from build123d import *

# Parameters (mm, degrees)
F0_R      = 30
F0_R_2    = 27.5
F1_DEPTH  = 38
F3_R      = 30
F3_R_2    = 27.5
F4_DEPTH  = 40
F6_W      = 24
F6_H      = 32
F7_DEPTH  = 65
F9_DEPTH  = 24
F10_DEPTH = 38
F12_DEPTH = 38
F13_R     = 4
F14_DEPTH = 38


with BuildPart() as f1:
    # F0 (on Front) → F1 (new body)
    with BuildSketch(Plane.XZ):
        with BuildLine():
            ThreePointArc((-32.5, 26.5), (-28.2573593129, 28.2573593129), (-26.5, 32.5))
            Line((-26.5, 32.5), (-28.5, 32.5))
            ThreePointArc((-28.5, 32.5), (-29.6715728753, 29.6715728753), (-32.5, 28.5))
            Line((-32.5, 28.5), (-32.5, 26.5))
        make_face()
        with BuildLine():
            Line((-28.5, 32.5), (-26.5, 32.5))
            ThreePointArc((-26.5, 32.5), (-36.7426406871, 36.7426406871), (-32.5, 26.5))
            Line((-32.5, 26.5), (-32.5, 28.5))
            ThreePointArc((-32.5, 28.5), (-35.3284271247, 35.3284271247), (-28.5, 32.5))
        make_face()
        with BuildLine():
            Line((26.5, 32.5), (-26.5, 32.5))
            ThreePointArc((-26.5, 32.5), (-28.2573593129, 28.2573593129), (-32.5, 26.5))
            Line((-32.5, 26.5), (-32.5, -26.5))
            ThreePointArc((-32.5, -26.5), (-28.2573593129, -28.2573593129), (-26.5, -32.5))
            Line((-26.5, -32.5), (26.5, -32.5))
            ThreePointArc((26.5, -32.5), (28.2573593129, -28.2573593129), (32.5, -26.5))
            Line((32.5, -26.5), (32.5, 26.5))
            ThreePointArc((32.5, 26.5), (28.2573593129, 28.2573593129), (26.5, 32.5))
        make_face()
        Circle(F0_R, mode=Mode.SUBTRACT)
        with BuildLine():
            ThreePointArc((38.5, 32.5), (32.5, 38.5), (26.5, 32.5))
            Line((26.5, 32.5), (28.5, 32.5))
            ThreePointArc((28.5, 32.5), (32.5, 36.5), (36.5, 32.5))
            ThreePointArc((36.5, 32.5), (35.3284271247, 29.6715728753), (32.5, 28.5))
            Line((32.5, 28.5), (32.5, 26.5))
            ThreePointArc((32.5, 26.5), (36.7426406871, 28.2573593129), (38.5, 32.5))
        make_face()
        with BuildLine():
            Line((28.5, 32.5), (26.5, 32.5))
            ThreePointArc((26.5, 32.5), (28.2573593129, 28.2573593129), (32.5, 26.5))
            Line((32.5, 26.5), (32.5, 28.5))
            ThreePointArc((32.5, 28.5), (29.6715728753, 29.6715728753), (28.5, 32.5))
        make_face()
        with BuildLine():
            ThreePointArc((-26.5, -32.5), (-28.2573593129, -28.2573593129), (-32.5, -26.5))
            Line((-32.5, -26.5), (-32.5, -28.5))
            ThreePointArc((-32.5, -28.5), (-29.6715728753, -29.6715728753), (-28.5, -32.5))
            Line((-28.5, -32.5), (-26.5, -32.5))
        make_face()
        with BuildLine():
            Line((-32.5, -28.5), (-32.5, -26.5))
            ThreePointArc((-32.5, -26.5), (-36.7426406871, -36.7426406871), (-26.5, -32.5))
            Line((-26.5, -32.5), (-28.5, -32.5))
            ThreePointArc((-28.5, -32.5), (-35.3284271247, -35.3284271247), (-32.5, -28.5))
        make_face()
        with BuildLine():
            ThreePointArc((38.5, -32.5), (36.7426406871, -28.2573593129), (32.5, -26.5))
            Line((32.5, -26.5), (32.5, -28.5))
            ThreePointArc((32.5, -28.5), (35.3284271247, -29.6715728753), (36.5, -32.5))
            ThreePointArc((36.5, -32.5), (32.5, -36.5), (28.5, -32.5))
            Line((28.5, -32.5), (26.5, -32.5))
            ThreePointArc((26.5, -32.5), (32.5, -38.5), (38.5, -32.5))
        make_face()
        with BuildLine():
            Line((32.5, -28.5), (32.5, -26.5))
            ThreePointArc((32.5, -26.5), (28.2573593129, -28.2573593129), (26.5, -32.5))
            Line((26.5, -32.5), (28.5, -32.5))
            ThreePointArc((28.5, -32.5), (29.6715728753, -29.6715728753), (32.5, -28.5))
        make_face()
        Circle(F0_R)
        Circle(F0_R_2, mode=Mode.SUBTRACT)
    extrude(amount=F1_DEPTH)

    # F3 (on offset) → F4 (join)
    with BuildSketch(Plane.XZ.offset(1)):
        Circle(F3_R)
        Circle(F3_R_2, mode=Mode.SUBTRACT)
    extrude(amount=-F4_DEPTH)

    # F6 (on offset) → F7 (join)
    with BuildSketch(Plane.XY.offset(-32.5)):
        with Locations((-44.5, -22)):
            Rectangle(F6_W, F6_H)
    extrude(amount=F7_DEPTH)

    # F8 (on face) → F9 (cut)
    with BuildSketch(Plane(origin=(-56.5, 0, 0), x_dir=(0, -1, 0), z_dir=(-1, 0, 0))):
        with BuildLine():
            Line((11.5996693186, -18.5), (6, -18.5))
            Line((6, -18.5), (6, -32.5))
            Line((6, -32.5), (19.7712382075, -32.5))
            ThreePointArc((19.7712382075, -32.5), (17.3473955456, -31.8732124062), (15.5312466875, -30.1499947))
            Line((15.5312466875, -30.1499947), (12.76000848, -25.716013568))
            ThreePointArc((12.76000848, -25.716013568), (12.1937562692, -24.4444314332), (12, -23.0660188679))
            Line((12, -23.0660188679), (12, -18.9003306814))
            ThreePointArc((12, -18.9003306814), (11.8827458581, -18.6172541419), (11.5996693186, -18.5))
        make_face()
        with BuildLine():
            ThreePointArc((28.4687533125, -30.1499947), (26.6526044544, -31.8732124062), (24.2287617925, -32.5))
            Line((24.2287617925, -32.5), (38, -32.5))
            Line((38, -32.5), (38, -18.5))
            Line((38, -18.5), (32.4003306814, -18.5))
            ThreePointArc((32.4003306814, -18.5), (32.1172541419, -18.6172541419), (32, -18.9003306814))
            Line((32, -18.9003306814), (32, -23.0660188679))
            ThreePointArc((32, -23.0660188679), (31.8062437308, -24.4444314332), (31.23999152, -25.716013568))
            Line((31.23999152, -25.716013568), (28.4687533125, -30.1499947))
        make_face()
        with BuildLine():
            Line((19.7712382075, 32.5), (6, 32.5))
            Line((6, 32.5), (6, 18.5))
            Line((6, 18.5), (11.5996693186, 18.5))
            ThreePointArc((11.5996693186, 18.5), (11.8827458581, 18.6172541419), (12, 18.9003306814))
            Line((12, 18.9003306814), (12, 23.0660188679))
            ThreePointArc((12, 23.0660188679), (12.1937562692, 24.4444314332), (12.76000848, 25.716013568))
            Line((12.76000848, 25.716013568), (15.5312466875, 30.1499947))
            ThreePointArc((15.5312466875, 30.1499947), (17.3473955456, 31.8732124062), (19.7712382075, 32.5))
        make_face()
        with BuildLine():
            Line((38, 32.5), (24.2287617925, 32.5))
            ThreePointArc((24.2287617925, 32.5), (26.6526044544, 31.8732124062), (28.4687533125, 30.1499947))
            Line((28.4687533125, 30.1499947), (31.23999152, 25.716013568))
            ThreePointArc((31.23999152, 25.716013568), (31.8062437308, 24.4444314332), (32, 23.0660188679))
            Line((32, 23.0660188679), (32, 18.9003306814))
            ThreePointArc((32, 18.9003306814), (32.1172541419, 18.6172541419), (32.4003306814, 18.5))
            Line((32.4003306814, 18.5), (38, 18.5))
            Line((38, 18.5), (38, 32.5))
        make_face()
    extrude(amount=-F9_DEPTH, mode=Mode.SUBTRACT)

    # F0 (on Front) → F10 (join)
    with BuildSketch(Plane.XZ):
        with BuildLine():
            ThreePointArc((38.5, 32.5), (32.5, 38.5), (26.5, 32.5))
            Line((26.5, 32.5), (28.5, 32.5))
            ThreePointArc((28.5, 32.5), (32.5, 36.5), (36.5, 32.5))
            ThreePointArc((36.5, 32.5), (35.3284271247, 29.6715728753), (32.5, 28.5))
            Line((32.5, 28.5), (32.5, 26.5))
            ThreePointArc((32.5, 26.5), (36.7426406871, 28.2573593129), (38.5, 32.5))
        make_face()
        with BuildLine():
            Line((-28.5, 32.5), (-26.5, 32.5))
            ThreePointArc((-26.5, 32.5), (-36.7426406871, 36.7426406871), (-32.5, 26.5))
            Line((-32.5, 26.5), (-32.5, 28.5))
            ThreePointArc((-32.5, 28.5), (-35.3284271247, 35.3284271247), (-28.5, 32.5))
        make_face()
        with BuildLine():
            ThreePointArc((38.5, -32.5), (36.7426406871, -28.2573593129), (32.5, -26.5))
            Line((32.5, -26.5), (32.5, -28.5))
            ThreePointArc((32.5, -28.5), (35.3284271247, -29.6715728753), (36.5, -32.5))
            ThreePointArc((36.5, -32.5), (32.5, -36.5), (28.5, -32.5))
            Line((28.5, -32.5), (26.5, -32.5))
            ThreePointArc((26.5, -32.5), (32.5, -38.5), (38.5, -32.5))
        make_face()
        with BuildLine():
            Line((-32.5, -28.5), (-32.5, -26.5))
            ThreePointArc((-32.5, -26.5), (-36.7426406871, -36.7426406871), (-26.5, -32.5))
            Line((-26.5, -32.5), (-28.5, -32.5))
            ThreePointArc((-28.5, -32.5), (-35.3284271247, -35.3284271247), (-32.5, -28.5))
        make_face()
    extrude(amount=F10_DEPTH)

    # F11 (on face) → F12 (cut)
    with BuildSketch(Plane(origin=(0, 0, 0), x_dir=(-1, 0, 0), z_dir=(0, 1, 0))):
        with BuildLine():
            Line((24.019457768, 32.5), (-24.019457768, 32.5))
            Line((-24.019457768, 32.5), (-17, 25.8134707125))
            Line((-17, 25.8134707125), (-15.2860959625, 25.8134707125))
            ThreePointArc((-15.2860959625, 25.8134707125), (0, 30), (15.2860959625, 25.8134707125))
            Line((15.2860959625, 25.8134707125), (17, 25.8134707125))
            Line((17, 25.8134707125), (24.019457768, 32.5))
        make_face()
        with BuildLine():
            Line((-17, -25.8134707125), (-24.019457768, -32.5))
            Line((-24.019457768, -32.5), (24.019457768, -32.5))
            Line((24.019457768, -32.5), (17, -25.8134707125))
            Line((17, -25.8134707125), (15.2860959625, -25.8134707125))
            ThreePointArc((15.2860959625, -25.8134707125), (0, -30), (-15.2860959625, -25.8134707125))
            Line((-15.2860959625, -25.8134707125), (-17, -25.8134707125))
        make_face()
    extrude(amount=-F12_DEPTH, mode=Mode.SUBTRACT)

    # F13 (on face) → F14 (cut)
    with BuildSketch(Plane.XZ.offset(38)):
        with Locations((-32.5, 32.5)):
            Circle(F13_R)
        with Locations((-32.5, -32.5)):
            Circle(F13_R)
    extrude(amount=-F14_DEPTH, mode=Mode.SUBTRACT)


solid = f1.part
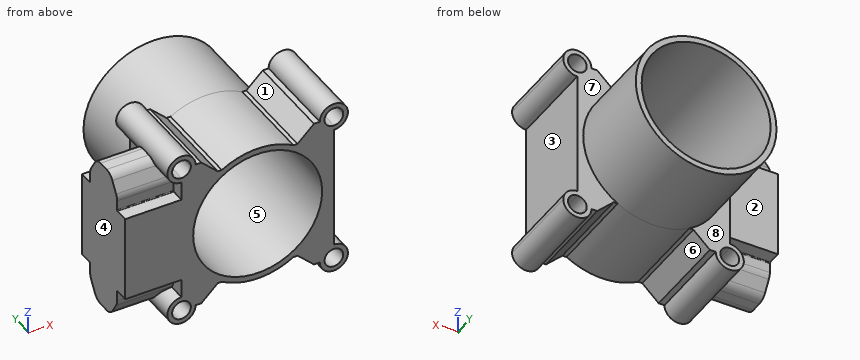
Read the model definition and answer for the solid it produces. Units are mm, in the model's axes. Face numbers are marked on the shaded views. A direction names the side the tool comes from. Round coordinates to 2 decimals unless told otherwise and drop trailing zeros. Order: outer loops, then holes, each group sorted by start corner. A loop starts at its lowest first (then second) coordinate and runs counter-clockwise, first axis right, second up.
1) The part is cut by section C-C on y = 21. Write down the section's boundary in (x, z).
2) Straight lines are drawn through the part: L1, parallel to Z at x = -32.5, y = -15; L2, parallel to Z at x = 0, y = 17; L3, parallel to Z at x = -44.5, y = -34. For each, find the intervals that lie inside material, in ascending order.
3) For the marked faces 5, 6, 7 and 8, determine the directions among +Z, -Z, +X, -X, +Y, -Y from which every point of the face is accessible in a straight line to the end or side of a thin tool.
4) Flat-ended cylindrical pins translate along their axes: pin 1 (4.5 mm diameter, centred on x = -38.5, y = -36, fed in from -Z); pin 2 (1.3 mm diameter, centred on x = -46, y = -22, fed in from +Z); pin 3 (0.5 mm diameter, centred on x = -16, y = -20, fed in from -Z). Find the tip coordinate at first contact, or state that the pin passes through.
5) The mould has two halves that part along X. Classify the marked faces 1, 2, 3 and 4: released by +X, released by -X, zero draft, split by the parting line, or undercut.
6) The part is cut by section B-B on z = -17. Write down the section's boundary in (x, y).
7) The part is cut by section A-A on x = 0. Write down the section's boundary in (y, z), plus the area to 3 significant figures.
8) The part is cut by section D-D on y = -22. Write down the section's boundary in (x, z), plus the area to 3 significant figures.
Resolved:
1. outline: circle Ø60 at (0, 0); hole circle Ø55 at (0, 0)
2. L1: z = -38.5 to -36.5, -28.5 to 28.5, 36.5 to 38.5
2. L2: z = -30 to -27.5, 27.5 to 30
2. L3: z = -18.5 to 18.5
3. face 5: +Y, -Y
3. face 6: -Z, +Y, -Y
3. face 7: +X, +Y
3. face 8: -X, +Y
4. pin 1: stops at z = -37.18
4. pin 2: stops at z = 32.5
4. pin 3: stops at z = -25.81
5. face 1: undercut
5. face 2: zero draft
5. face 3: released by +X
5. face 4: released by -X
6. outline: (-56.5, -38) - (-21.62, -38) - (-21.62, 39) - (-24.72, 39) - (-24.72, 0) - (-32.5, 0) - (-32.5, -6) - (-56.5, -6) - close; (21.62, -38) - (32.5, -38) - (32.5, 0) - (24.72, 0) - (24.72, 39) - (21.62, 39) - close
7. outline: (-38, -30) - (39, -30) - (39, -27.5) - (-38, -27.5) - close; (-38, 27.5) - (39, 27.5) - (39, 30) - (-38, 30) - close
7. area: 385 mm2
8. outline: (-56.5, -32.5) - (-38.5, -32.5) arc R6 ccw to (-26.5, -32.5) - (-24.02, -32.5) - (-17, -25.81) - (-15.29, -25.81) arc R30 ccw to (15.29, -25.81) - (17, -25.81) - (24.02, -32.5) - (26.5, -32.5) arc R6 ccw (long way) to (32.5, -26.5) - (32.5, 26.5) arc R6 ccw (long way) to (26.5, 32.5) - (24.02, 32.5) - (17, 25.81) - (15.29, 25.81) arc R30 ccw to (-15.29, 25.81) - (-17, 25.81) - (-24.02, 32.5) - (-26.5, 32.5) arc R6 ccw to (-38.5, 32.5) - (-56.5, 32.5) - close; hole circle Ø8 at (-32.5, -32.5); hole circle Ø8 at (-32.5, 32.5); hole circle Ø55 at (0, 0); hole circle Ø8 at (32.5, -32.5); hole circle Ø8 at (32.5, 32.5)
8. area: 3,120 mm2
